Geometry check sheet. Reference: the model listing, model coordinates, mm. A direction names the side the tool comes from. Round coordinates to 2 decimals unless told otherwise and drop trailing zeros. Order: outer loops, then holes, each group sorted by start corner. A loop starts at its lowest first (then second) coordinate and runs counter-clockwise, first axis right, second up.
(1) Sectioned sample at C-C (y = 6). Record the boundary of the cut face in (x, z).
(2) Material ranges on line 1 along X through (y, z) = (2.1, 56.5); line 2 along Z through (x, y) = (-86.5, 1.2); line 3 along Z through (x, y) = (-54.5, 22), recorded low to high.
(3) Sectioned sample at B-B (x = -35.5). Record the boundary of the cut face in (y, z), plus the area to 3 significant figures.
(4) Sectioned sample at D-D (z = 1.5). Record the boundary of the cut face in (x, y).
(5) Release check for a two-part mould opening along Z. For faces 4 (the face through (-88.007, 2.028, -55.345)), 5 (the face through (84.603, 2.028, 56.417)), 6 (the face through (-1, 14, -50.7)), 7 (the face through (93.49, 2.03, 63.65)) record: +Z half, -Z half, draft (parallel to the pull), parting line (faces both ways), or undercut.
(6) Sectioned sample at A-A (x = 0). Record the boundary of the cut face in (y, z), plus the area to 3 significant figures.
(7) Go/stop test with flat-tipped pins: pin 1 (5 mm diameter, centred on y = 17.5, z = -40.5, fed in from +X); pin 2 (3 mm diameter, centred on x = 17.5, y = 7.5, fed in from -Z); pin 3 (10 mm diameter, centred on y = 15.5, z = 0.5, fed in from -X). Record where each tip stops, or that it passes through.
(8) Set-up check for faces 1 (the face through (-80.7, 14, 1)), 2 (the face through (80.7, 14, 1)), 3 (the face through (-52, 4, -1)): record each of +Z, -Z, +X, -X, +Y, -Y from which the full face is reachable in a straight line by a thin tool's end or side.
from build123d import *

# Parameters (mm, degrees)
SKETCH1_W                    = 193
SKETCH1_H                    = 133
BOSS_EXTRUDE1_DEPTH          = 4
SKETCH2_W                    = 161.4
SKETCH2_H                    = 101.4
SKETCH2_W_2                  = 153.4
SKETCH2_H_2                  = 93.4
EXTRUDE_THIN1_DEPTH          = 20
SKETCH3_W                    = 112
SKETCH3_H                    = 70.9
CUT_EXTRUDE3_DEPTH           = 15
FILLET1_R                    = 1
F_25_0_1495_DIAMETER_HOLE2_D = 3.7973
FILLET3_R                    = 10
TAP_DRILL_FOR_6_32_TAP1_D    = 2.7051


with BuildPart() as part:
    # Sketch1 → Boss-Extrude1 (new body)
    with BuildSketch(Plane(origin=(0, 0, 0), x_dir=(1, 0, 0), z_dir=(0, 1, 0))):
        Rectangle(SKETCH1_W, SKETCH1_H)
    extrude(amount=BOSS_EXTRUDE1_DEPTH)

    # Sketch2 → Extrude-Thin1 (add)
    with BuildSketch(Plane(origin=(0, 4, 0), x_dir=(1, 0, 0), z_dir=(0, 1, 0))):
        Rectangle(SKETCH2_W, SKETCH2_H)
        Rectangle(SKETCH2_W_2, SKETCH2_H_2, mode=Mode.SUBTRACT)
    extrude(amount=EXTRUDE_THIN1_DEPTH)

    # Sketch3 → Cut-Extrude3 (cut)
    with BuildSketch(Plane.XZ):
        with Locations((4.45, -3.25)):
            Rectangle(SKETCH3_W, SKETCH3_H)
    extrude(amount=-CUT_EXTRUDE3_DEPTH, mode=Mode.SUBTRACT)

    # Fillet1
    fillet1_edges = [part.edges().sort_by_distance(p)[0] for p in [
        (60.45, 0, -3.25),
        (4.45, 0, 32.2),
        (-51.55, 0, -3.25),
        (4.45, 0, -38.7),
    ]]
    fillet(fillet1_edges, radius=FILLET1_R)

    # #25 (0.1495) Diameter Hole2 (through all)
    with Locations(Plane(origin=(0, 0, 0), x_dir=(-1, 0, 0), z_dir=(0, -1, 0))):
        with Locations((86.5, -56.5), (86.5, 56.5), (-86.5, 56.5), (-86.5, -56.5), (0, -56.5), (0, 56.5)):
            Hole(F_25_0_1495_DIAMETER_HOLE2_D / 2)

    # Fillet3
    fillet3_edges = [part.edges().sort_by_distance(p)[0] for p in [
        (96.5, 2, 66.5),
        (-96.5, 2, 66.5),
        (-96.5, 2, -66.5),
        (96.5, 2, -66.5),
    ]]
    fillet(fillet3_edges, radius=FILLET3_R)

    # Tap Drill for #6-32 Tap1 (through all)
    with Locations(Plane.ZY.offset(80.7)):
        with Locations((-40.7, 14), (40.7, 14)):
            Hole(TAP_DRILL_FOR_6_32_TAP1_D / 2)


solid = part.part
Answer below:
1. outline: (-80.7, -50.7) - (80.7, -50.7) - (80.7, 50.7) - (-80.7, 50.7) - close; hole (-76.7, -46.7) - (76.7, -46.7) - (76.7, 46.7) - (-76.7, 46.7) - close
2. line 1: x = -96.5 to -88.4, -84.6 to -1.9, 1.9 to 84.6, 88.4 to 96.5
2. line 2: z = -66.5 to -58.4, -54.6 to 54.6, 58.4 to 66.5
2. line 3: z = -50.7 to -46.7, 46.7 to 50.7
3. outline: (0, -66.5) - (4, -66.5) - (4, -50.7) - (24, -50.7) - (24, -46.7) - (4, -46.7) - (4, -38.7) - (1, -38.7) arc R1 ccw to (0, -39.7) - close; (0, 33.2) arc R1 ccw to (1, 32.2) - (4, 32.2) - (4, 46.7) - (24, 46.7) - (24, 50.7) - (4, 50.7) - (4, 66.5) - (0, 66.5) - close
3. area: 408 mm2
4. outline: (-96.5, 0) - (-52.55, 0) arc R1 ccw to (-51.55, 1) - (-51.55, 4) - (-76.7, 4) - (-76.7, 24) - (-80.7, 24) - (-80.7, 4) - (-96.5, 4) - close; (60.45, 1) arc R1 ccw to (61.45, 0) - (96.5, 0) - (96.5, 4) - (80.7, 4) - (80.7, 24) - (76.7, 24) - (76.7, 4) - (60.45, 4) - close
5. face 4: undercut
5. face 5: undercut
5. face 6: -Z half
5. face 7: +Z half
6. outline: (0, -66.5) - (4, -66.5) - (4, -58.4) - (0, -58.4) - close; (0, -54.6) - (4, -54.6) - (4, -50.7) - (24, -50.7) - (24, -46.7) - (4, -46.7) - (4, -38.7) - (1, -38.7) arc R1 ccw to (0, -39.7) - close; (0, 33.2) arc R1 ccw to (1, 32.2) - (4, 32.2) - (4, 46.7) - (24, 46.7) - (24, 50.7) - (4, 50.7) - (4, 54.6) - (0, 54.6) - close; (0, 58.4) - (4, 58.4) - (4, 66.5) - (0, 66.5) - close
6. area: 378 mm2
7. pin 1: stops at x = 80.7
7. pin 2: stops at z = -50.7
7. pin 3: stops at x = -80.7
8. face 1: +Z, -Z, -X, +Y
8. face 2: +Z, -Z, +X, +Y
8. face 3: +Y
